The model under review builds one solid part; all positions refer to its coordinate system, in mm. Face numbers are marked on the shaded views. A direction names the side the tool comes from. Round coordinates to 2 decimals unless told otherwise and drop trailing zeros. Order: outer loops, then holes, each group sorted by start corner. A loop starts at its lowest first (then second) coordinate and runs counter-clockwise, first axis right, second up.
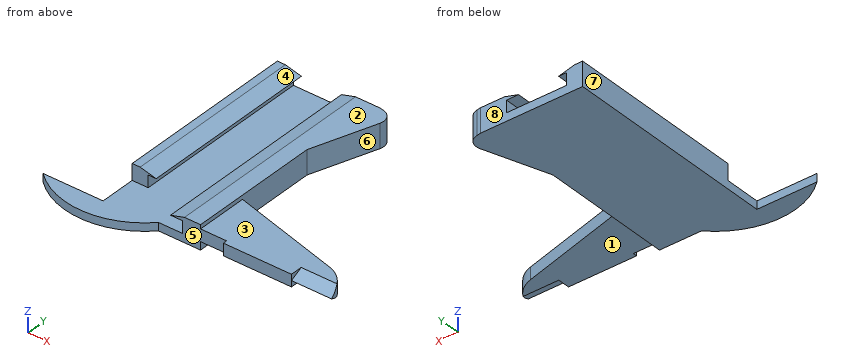
```python
from build123d import *

# Parameters (mm, degrees)
F1_DEPTH  = 53
F3_DEPTH  = 3
F6_DEPTH  = 10
F8_DEPTH  = 2
F9_W      = 4
F9_H      = 8
F9_W_2    = 2
F10_DEPTH = 4
F12_DEPTH = 6
F13_R     = 3


with BuildPart() as f1:
    # F0 (on Front) → F1 (new body)
    with BuildSketch(Plane.XZ):
        Polygon((0, 3), (0, 0), (-15, 0), (-15, 3), (-13, 3), (-17, 4), (-19, 4), (-19, -2), (4.5, -2), (4.5, 4), (0.5, 4), (-3, 3), align=None)
    extrude(amount=F1_DEPTH)

    # F2 (on Top) → F3 (join)
    with BuildSketch(Plane.XY):
        with BuildLine():
            Line((32.151714, -47.409254), (4.5, -40))
            Line((4.5, -40), (4.5, -53))
            Line((4.5, -53), (11, -53))
            Line((11, -53), (11, -54))
            Line((11, -54), (38, -54))
            ThreePointArc((38, -54), (36.065012, -49.826902), (32.151714, -47.409254))
        make_face()
    extrude(amount=F3_DEPTH)

    # F5 (on offset) → F6 (cut)
    with BuildSketch(Plane.YZ.offset(38)):
        Polygon((-59, 3), (-59, 0), (-51, 0), (-54, 1.5), (-51, 3), align=None)
    extrude(amount=-F6_DEPTH, mode=Mode.SUBTRACT)

    # F7 (on face) → F8 (join)
    with BuildSketch(Plane(origin=(0, 0, -2), x_dir=(1, 0, 0), z_dir=(0, 0, -1))):
        with BuildLine():
            Line((-19, 54), (-19, 53))
            Line((-19, 53), (-6, 53))
            ThreePointArc((-6, 53), (-19.795634, 59.222249), (-34, 54))
            Line((-34, 54), (-19, 54))
        make_face()
    extrude(amount=-F8_DEPTH)

    # F9 (on face) → F10 (cut)
    with BuildSketch(Plane.XY.offset(4)):
        with Locations((-15, -49)):
            Rectangle(F9_W, F9_H)
        with Locations((-18, -49)):
            Rectangle(F9_W_2, F9_H)
    extrude(amount=-F10_DEPTH, mode=Mode.SUBTRACT)

    # F11 (on face) → F12 (join)
    with BuildSketch(Plane.XY.offset(4)):
        Polygon((4.5, 0), (4.5, -20), (11, -0.793471), (6.5, 0), align=None)
    extrude(amount=-F12_DEPTH)

    # F13
    f13_edges = [f1.edges().sort_by_distance(p)[0] for p in [
        (11, -0.793471, 1),
    ]]
    fillet(f13_edges, radius=F13_R)


solid = f1.part
```
(1) Draft analysis for pull direction Y (two halves, no side actions). For the marked faces 6, 7 and 8, state which applies: pulls with the +Y half, pulls with the -Y half, needs draft (parallel to the pull), parting line crosses it, or undercut.
Data:
face 6: undercut
face 7: needs draft
face 8: pulls with the +Y half
(2) To check wall thickness, follow probe 1 along X at (y, z) = (-37, 2.7); probe 2 along Z at (x, y) = (-20, -56); probe 3 along X at (y, z) = (-16.5, 0.9). State the ranges of each line that lie inside material, in increasing order.
Data:
probe 1: x = -19 to -15, 0 to 4.5
probe 2: z = -2 to 0
probe 3: x = -19 to -15, 0 to 5.68
(3) For the marked faces 1, 2, 3, 4 and 5, list the 3-axis set-ups (+Z, -Z, +X, -X, +Y, -Y) from which the entire face can be reached by the end or side of a thin tool; tool diameter is ignored.
Data:
face 1: -Z, +X, -Y
face 2: +Z, +X, -X, +Y, -Y
face 3: +Z, +X, -Y
face 4: +Z, +Y, -Y
face 5: +Z, -Z, -Y
(4) Consider section B-B (x = -8). Write out the cut boundary in (y, z), and give its area (3 significant figures).
Data:
outline: (-54.84, -2) - (0, -2) - (0, 0) - (-54.84, 0) - close
area: 110 mm2
(5) Consider section A-A (y = -31). Write out the cut boundary in (x, z).
Data:
outline: (-19, -2) - (4.5, -2) - (4.5, 4) - (0.5, 4) - (-3, 3) - (0, 3) - (0, 0) - (-15, 0) - (-15, 3) - (-13, 3) - (-17, 4) - (-19, 4) - close
(6) Insertion check: pin 1 (3 mm diameter, centred on y = -9.5, z = 0, fed in from +X); pin 2 (1.2 mm diameter, centred on y = -52.5, z = 2, fed in from +X); pin 3 (7 mm diameter, centred on x = 15.5, y = -49, fed in from +Z). Each pin has a flat end and moves straight along its axis. Give the tip position at first contact, or say it passes through.
Data:
pin 1: stops at x = 8.56
pin 2: stops at x = 37.82
pin 3: stops at z = 3
(7) Consider section C-C (y = -15.5). Write out the cut boundary in (x, z).
Data:
outline: (-19, -2) - (6.02, -2) - (6.02, 4) - (0.5, 4) - (-3, 3) - (0, 3) - (0, 0) - (-15, 0) - (-15, 3) - (-13, 3) - (-17, 4) - (-19, 4) - close
(8) Consider section D-D (x = 23). Write out the cut boundary in (y, z), and give its area (3 significant figures).
Data:
outline: (-54, 0) - (-44.96, 0) - (-44.96, 3) - (-54, 3) - close
area: 27.1 mm2
